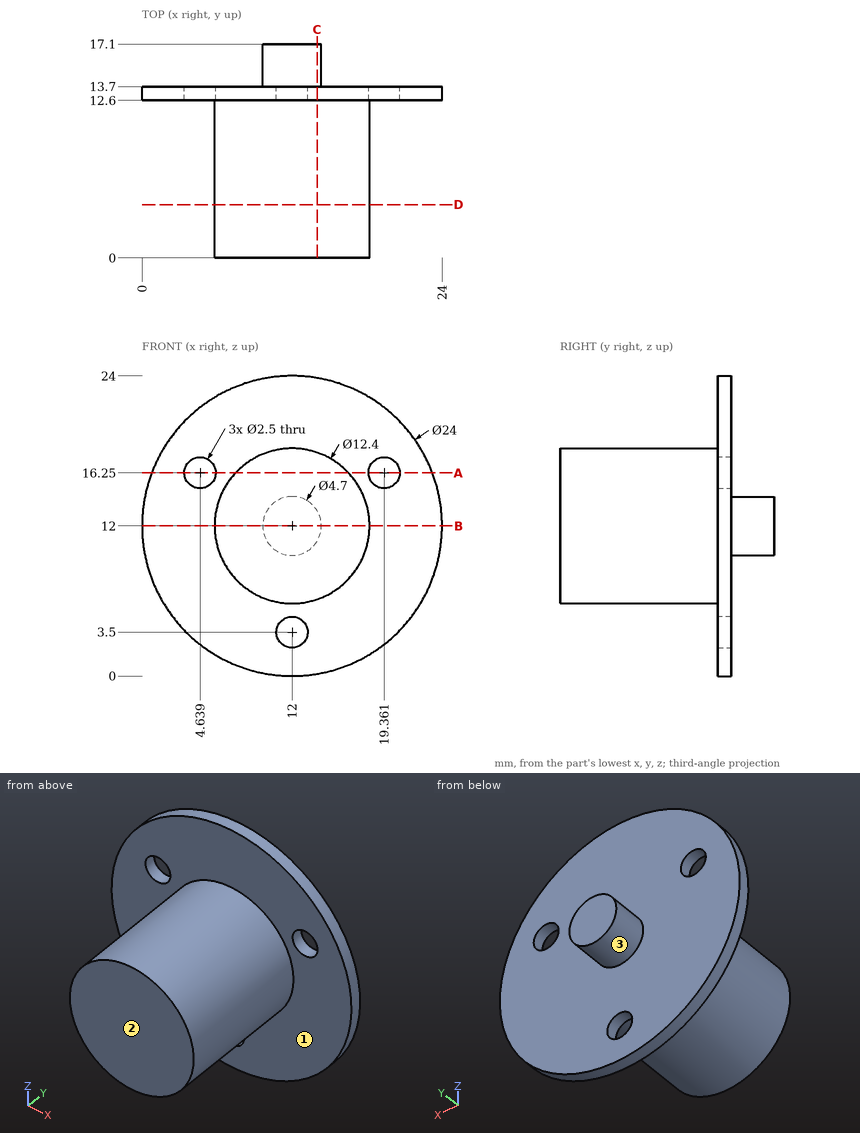
Source: three-view drawing plus pictorial views. Frame: mm from the lowest corner of the part. A direction names the side the tool comes from. Round coordinates to 2 decimals unless told otherwise and drop trailing zeros. Order: outer loops, then holes, each group sorted by start corner. A loop starts at its lowest first (then second) coordinate and runs counter-clockwise, first axis right, second up. Notation, with made-up numbers: M 64.5,73.25 L 76.5,73.25 A21 ccw 76.5,84.25 Z; hole C -37,86 d5. An arc over 180 degrees is marked long. One line per item, written item: value.
(1) Line query: probe 1 along X at (y, z) = (12.9, 16.25); probe 2 along Y at (x, z) = (14.5, 11.5); probe 3 along Y at (x, z) = (7.25, 7.5). Output: solid intervals per line, ascending. Write a range as [from, to].
Result sheet:
probe 1: [0.78, 3.39], [5.89, 18.11], [20.61, 23.22]
probe 2: [0, 13.7]
probe 3: [12.6, 13.7]
(2) Reachability of the marked faces 1, 2 and 3 from +Z, -Z, +X, -X, +Y, -Y: full face, straight path, thin tool, end or side. Return the list, or none.
Result sheet:
face 1: -Y
face 2: +Z, -Z, +X, -X, -Y
face 3: +Y
(3) Cut plane A-A (z = 16.25). Return the cut outline in (x, y).
Result sheet:
outline: M 0.78,12.6 L 3.39,12.6 L 3.39,13.7 L 0.78,13.7 Z; M 5.89,12.6 L 7.49,12.6 L 7.49,0 L 16.51,0 L 16.51,12.6 L 18.11,12.6 L 18.11,13.7 L 5.89,13.7 Z; M 20.61,12.6 L 23.22,12.6 L 23.22,13.7 L 20.61,13.7 Z
(4) Cut plane D-D (y = 4.25). Return the cut outline in (x, z).
Result sheet:
outline: C 12,12 d12.4
(5) Cut plane B-B (z = 12). Return the cut outline in (x, y), and give its area (3 significant figures).
Result sheet:
outline: M 0,12.6 L 5.8,12.6 L 5.8,0 L 18.2,0 L 18.2,12.6 L 24,12.6 L 24,13.7 L 14.35,13.7 L 14.35,17.1 L 9.65,17.1 L 9.65,13.7 L 0,13.7 Z
area: 199 mm2
(6) Pin query (flat end, axial travel): P1, Ø2, axis at x = 4.64, z = 16.25, coming from the +Y side; P2, Ø4, axis at x = 13.5, z = 7.5, coming from the +Y side; P3, Ø8, axis at x = 21, z = 4.5, coming from the -Y side; P4, Ø10, axis at y = 2, z = 5, coming from the +X side. Return the tip coordinate at first contact, or that it passes through.
Result sheet:
P1: through
P2: y = 13.7
P3: y = 12.6
P4: x = 17.87
(7) Cut plane C-C (x = 14). Return the cut outline in (y, z), and give its area (3 significant figures).
Result sheet:
outline: M 0,6.13 L 12.6,6.13 L 12.6,0.17 L 13.7,0.17 L 13.7,10.77 L 17.1,10.77 L 17.1,13.23 L 13.7,13.23 L 13.7,23.83 L 12.6,23.83 L 12.6,17.87 L 0,17.87 Z
area: 182 mm2
